Autodesk Inventor part; units mm, degrees
ref_plane "YZ Plane" through (0, 0, 0) normal (1, 0, 0) x (0, 1, 0)
ref_plane "XZ Plane" through (0, 0, 0) normal (0, 1, 0) x (-1, 0, 0)
ref_plane "XY Plane" through (0, 0, 0) normal (0, 0, 1) x (1, 0, 0)
sketch "Sketch1" plane through (0, 0, 0) normal (0, 0, 1) x (1, 0, 0)
  circle A0 centre (0, 0) radius 25.4
  line L0 (7.9189, 0) -> (3.9595, -6.858)
  line L1 (3.9595, -6.858) -> (-3.9595, -6.858)
  line L2 (-3.9595, -6.858) -> (-7.9189, 0)
  line L3 (-7.9189, 0) -> (-3.9595, 6.858)
  line L4 (-3.9595, 6.858) -> (3.9595, 6.858)
  line L5 (3.9595, 6.858) -> (7.9189, 0)
  dimension "d0" = 50.8
  dimension "d1" = 13.716
extrude "Extrusion1" add sketch "Sketch1" along normal mid plane 76.2
sketch "Sketch3" plane through (0, 0, 0) normal (1, 0, 0) x (0, 1, 0)
  line L0 (25.4, 38.1) -> (-25.4, 38.1)
  line L1 (25.4, 38.1) -> (38.1, 38.1)
  line L2 (25.4, -38.1) -> (25.4, 38.1)
  line L3 (0, -53.34) -> (0, 53.34)
  line L4 (38.1, 38.1) -> (38.1, 12.7)
  line L5 (38.1, 12.7) -> (24.2886, 6.2597)
  line L6 (24.2886, 6.2597) -> (25.4, 6.7779)
  line L7 (25.4, -38.1) -> (25.4, 38.1)
  point P0 (0, 0)
  point P1 (25.4, 19.4779)
  point P2 (25.4, 6.7779)
  dimension "d9" = 12.7
  dimension "d12" = 25.4
  dimension "d13" = 115
revolve "Revolution1" add sketch "Sketch3" angle 360 about axis through (0, 0, -10) along (0, 0, 1)
sketch "Sketch4" plane through (0, 0, 0) normal (1, 0, 0) x (0, 1, 0)
  line L0 (25.4, -38.1) -> (25.4, 6.7779)
  line L1 (-25.4, -38.1) -> (25.4, -38.1)
  line L2 (25.4, -38.1) -> (38.1, -38.1)
  line L3 (38.1, -38.1) -> (38.1, -31.75)
  line L4 (38.1, -31.75) -> (24.8707, -25.5811)
  line L5 (0, -46.9275) -> (0, 14.8652)
  line L6 (24.8707, -25.5811) -> (25.4, -25.8279)
  line L7 (25.4, -38.1) -> (25.4, 6.7779)
  point P0 (0, 0)
  point P1 (25.4, -25.8279)
  dimension "d14" = 12.7
  dimension "d15" = 6.35
  dimension "d16" = 115
revolve "Revolution2" add sketch "Sketch4" angle 360 about axis through (0, 0, -10) along (0, 0, 1)
properties part number "pulley"
CAD build for the part. Positions are in the model's coordinates, mm. A direction names the side the tool comes from. Round coordinates to 2 decimals unless told otherwise and drop trailing zeros. Write each loop counter-clockwise with the first axis right and the second up, starting at its lowest first coordinate (ties: lowest second). Pieces come first, ordered by that corner, then holes. Notation, with made-up numbers: (-17.75, 80) - (-0.75, 80) arc R16 ccw to (-0.75, 109) - close; hole circle Ø8 at (-29, 16.5). An arc over 180 degrees is marked (long way). Return JSON: item names as keys, results as strings. Group by question number.
Item 1: 3-axis set-ups, long thin cutter, end or side, ignore diameter. For faces 1 (the face through (0, -6.858, -1)), 2 (the face through (-25.57, -5.68, -26.2)), 3 (the face through (8, 1, -38.1)): which of +Z, -Z, +X, -X, +Y, -Y reach the whole face in a straight line?
Item 2: Flat gauge pins, fed straight in: pin 1 Ø2 at (x, z) = (28, -11.5) entering from +Y; pin 2 Ø4 at (x, z) = (1.5, -6.5) entering from +Y; pin 3 Ø2 at (y, z) = (-27, 26) entering from +X; pin 4 Ø2.5 at (x, z) = (0.5, -10) entering from -Y. Where does each tip first touch, or does it go through?
Item 3: Band-saw the part on C-C on z = 18.5. List the corners of the cut face in (x, y).
Item 4: Mould opens along Y. For faces 4 (the face through (-1, 8, 38.1)), 5 (the face through (-5.506, -24.796, -9.297)), 6 (the face through (-5.9, -3.5, -0.5)) say: +Y half, -Y half, draft (parallel to the pull), parting line (faces both ways), or undercut.
Item 5: Probe probe 1 along X at (y, z) = (0, 10); probe 2 along Z at (x, y) = (25, -22); probe 3 along Z at (x, y) = (4, -33). List the from-to ranges inside material, lowest first.
Item 6: Band-saw the part on A-A on z = -17.5. List the corners of the cut face in (x, y), plus the area to 3 significant figures.
Item 7: Band-saw the part on B-B on x = 0. List the corners of the cut face in (y, z).
Resolved:
{
 "1": {"face 1": "+Z, -Z", "face 2": "none", "face 3": "-Z, +X, -X, +Y, -Y"},
 "2": {"pin 1": "passes through", "pin 2": "stops at y = 25.4", "pin 3": "stops at x = 27.85", "pin 4": "stops at y = -25.4"},
 "3": {"outline": "circle Ø76.2 at (0, 0); hole (-7.92, 0) - (-3.96, -6.86) - (3.96, -6.86) - (7.92, 0) - (3.96, 6.86) - (-3.96, 6.86) - close"},
 "4": {"face 4": "draft", "face 5": "parting line", "face 6": "undercut"},
 "5": {"probe 1": "x = -32.31 to -7.92, 7.92 to 32.31", "probe 2": "z = -38.1 to -29.51, 10.46 to 38.1", "probe 3": "z = -38.1 to -29.48, 10.43 to 38.1"},
 "6": {"outline": "circle Ø50.8 at (0, 0); hole (-7.92, 0) - (-3.96, -6.86) - (3.96, -6.86) - (7.92, 0) - (3.96, 6.86) - (-3.96, 6.86) - close", "area": "1,860 mm²"},
 "7": {"outline": "(-38.1, -38.1) - (-6.86, -38.1) - (-6.86, 38.1) - (-38.1, 38.1) - (-38.1, 12.7) - (-25.4, 6.78) - (-25.4, -25.83) - (-38.1, -31.75) - close; (6.86, -38.1) - (38.1, -38.1) - (38.1, -31.75) - (25.4, -25.83) - (25.4, 6.78) - (38.1, 12.7) - (38.1, 38.1) - (6.86, 38.1) - close"}
}
